Build history of the part. All positions in model axes, mm. Face numbers are marked on the shaded views. A direction names the side the tool comes from. Round coordinates to 2 decimals unless told otherwise and drop trailing zeros. Write each loop counter-clockwise with the first axis right and the second up, starting at its lowest first coordinate (ties: lowest second). Pieces come first, ordered by that corner, then holes.
Item 1: Wall check: probe 1 along Z at (x, y) = (-131.75, -5); probe 2 along X at (y, z) = (-3, 2). Give the ranges that are in metal, low to high.
Item 2: 3-axis set-ups, long thin cutter, end or side, ignore diameter. For the marked faces 1 and 2: which of +Z, -Z, +X, -X, +Y, -Y reach the whole face in a straight line?
Item 3: Band-saw the part on D-D, the plane x = -37.5. Write the cut outline in (y, z).
Item 4: Band-saw the part on B-B, the plane y = -5. Write the cut outline in (x, z), then the cut area to 3 significant figures.
Item 5: Band-saw the part on A-A, the plane z = 5. Write the cut outline in (x, y).
Item 6: Band-saw the part on C-C, the plane y = 5. Write the cut outline in (x, z).
Item 7: Drop flat-ended pins along their axis: pin 1 Ø2 at (y, z) = (-4, 9) entering from +X; pin 2 Ø1.8 at (y, z) = (5, 4) entering from +X; pin 3 Ø3 at (x, z) = (-77, 1.5) entering from -Y. Give the stop position or say it passes through.
```python
from build123d import *

# Parameters (mm, degrees)
BOSS_EXTRUDE1_DEPTH = 10
SKETCH4_R           = 3
CUT_EXTRUDE2_DEPTH  = 150
SKETCH4_3_R         = 3
CUT_EXTRUDE3_DEPTH  = 20


with BuildPart() as part:
    # Sketch1 → Boss-Extrude1 (new body)
    with BuildSketch(Plane.XY):
        Polygon((-140, 10), (0, 10), (0, 0), (-130, 0), (-130, -10), (-140, -10), align=None)
    extrude(amount=BOSS_EXTRUDE1_DEPTH)

    # Sketch4 → Cut-Extrude2 (cut)
    with BuildSketch(Plane(origin=(0, 0, 0), x_dir=(0, 0, -1), z_dir=(1, 0, 0))):
        with Locations(Location((-5, -5, 0), (0, 0, 90))):
            Circle(SKETCH4_R)
    extrude(amount=-CUT_EXTRUDE2_DEPTH, mode=Mode.SUBTRACT)

    # Sketch4_3 → Cut-Extrude3 (cut)
    with BuildSketch(Plane(origin=(0, 0, 0), x_dir=(0, 0, -1), z_dir=(1, 0, 0))):
        with Locations((-5, 5)):
            Circle(SKETCH4_3_R)
    extrude(amount=-CUT_EXTRUDE3_DEPTH, mode=Mode.SUBTRACT)


solid = part.part
```
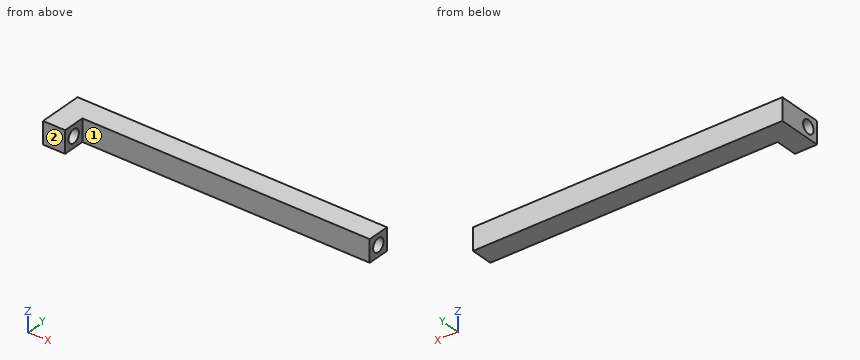
Results:
1. probe 1: z = 0 to 2, 8 to 10
1. probe 2: x = -140 to -130
2. face 1: +Z, -Z, +X, -Y
2. face 2: +Z, -Z, +X, -X, -Y
3. outline: (0, 0) - (10, 0) - (10, 10) - (0, 10) - close
4. outline: (-140, 0) - (-130, 0) - (-130, 2) - (-140, 2) - close; (-140, 8) - (-130, 8) - (-130, 10) - (-140, 10) - close
4. area: 40.0 mm2
5. outline: (-140, -10) - (-130, -10) - (-130, -8) - (-140, -8) - close; (-140, -2) - (-130, -2) - (-130, 0) - (0, 0) - (0, 2) - (-20, 2) - (-20, 8) - (0, 8) - (0, 10) - (-140, 10) - close
6. outline: (-140, 0) - (0, 0) - (0, 2) - (-20, 2) - (-20, 8) - (0, 8) - (0, 10) - (-140, 10) - close
7. pin 1: stops at x = -130
7. pin 2: stops at x = -20
7. pin 3: stops at y = 0
